CAD build for the part. Positions are in the model's coordinates, mm. Face numbers are marked on the shaded views. A direction names the side the tool comes from. Coordinates: 2 decimals unless noted, no trailing zeros. Loops run counter-clockwise (first coordinate to the right, second up) from the corner with the lowest first, then second, coordinate; pieces in that order, holes last. Notation, with made-up numbers: (4, -3) -> (21, -3) arc R27 cw to (21, 27) -> close; hole circle Ø4 at (77, 86). An arc over 180 degrees is marked (long way). Return JSON: item names as keys, results as strings. Group by question number.
(1) Flat gauge pins, fed straight in: pin 1 Ø0.8 at (y, z) = (-199, 56.5) entering from +X; pin 2 Ø0.5 at (x, z) = (150.5, 36) entering from -Y; pin 3 Ø6 at (x, z) = (86, 46) entering from -Y; pin 4 Ø1.1 at (y, z) = (0.5, 36) entering from -X. Where does each tip first touch, or does it go through?
(2) Saw through at D-D on x = -201. Write the cut outline in (y, z), then the cut area to 3 significant figures.
(3) Saw through at C-C on y = 153. Write the cut outline in (x, z), then the cut area to 3 significant figures.
(4) Saw through at A-A on z = 51.5. Write the cut outline in (x, y), then the cut area to 3 significant figures.
(5) Saw through at B-B on x = -31. Write the cut outline in (y, z).
(6) Probe L1, parallel to Y at x = -49.5, z = 43.25; L2, parallel to Y at x = -190, z = 54; L3, parallel to Z at x = -160.5, y = 91. List the from-to ranges inside material, lowest first.
(7) Tool access for the marked faces 5 and 6: list every direction of +Z, -Z, +X, -X, +Y, -Y with a clear straight run to the whole face (end or side of a thin tool).
(8) Mould opens along Y. For the marked faces 1, 2, 3 and 4 say: pulls with the +Y half, pulls with the -Y half, needs draft (parallel to the pull), parting line crosses it, or undercut.
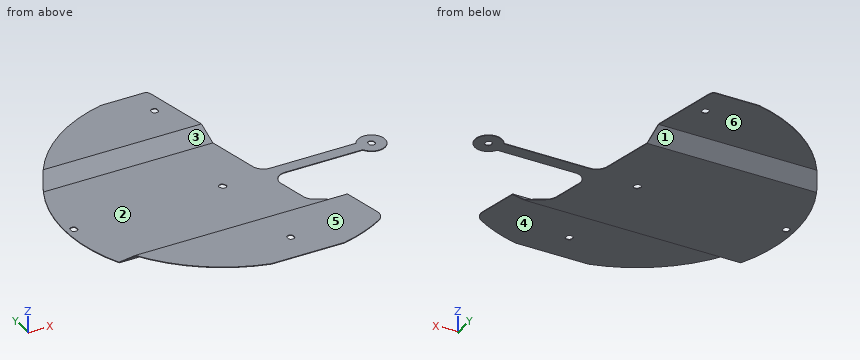
```python
from build123d import *

# Parameters (mm, degrees)
SALIENTE_EXTRUIR1_DEPTH    = 271
CORTAR_EXTRUIR6_DEPTH      = 372.705950862
CORTAR_EXTRUIR6_DEPTH_BACK = 372.705950862
CROQUIS2_W                 = 769.435607064
CROQUIS2_H                 = 651.661171996
CORTAR_EXTRUIR9_DEPTH      = 367.633759911
CORTAR_EXTRUIR9_DEPTH_BACK = 367.633759911


with BuildPart() as part:
    # Croquis1 → Saliente-Extruir1 (new, symmetric)
    with BuildSketch(Plane(origin=(0, 0, 0), x_dir=(0, 0, -1), z_dir=(1, 0, 0))):
        Polygon((-36.5, -110), (-36.5, 110), (-56.747809705, 134.130399958), (-56.747809705, 248), (-55.747809705, 248), (-55.747809705, 134.494370193), (-35.5, 110.363970234), (-35.5, -110.363970234), (-55.747809705, -134.494370193), (-55.747809705, -248), (-56.747809705, -248), (-56.747809705, -134.130399958), align=None)
    extrude(amount=SALIENTE_EXTRUIR1_DEPTH, both=True)

    # Croquis2 → Cortar-Extruir6 (cut, two sides: drawn at the far end of the back side and taken through both)
    with BuildSketch(Plane.XY.offset(-CORTAR_EXTRUIR6_DEPTH_BACK)):
        Rectangle(CROQUIS2_W, CROQUIS2_H)
        with BuildLine():
            ThreePointArc((18.264078831, 239.138091094), (11.247490428, 250.568826506), (-1.413221116, 254.996083903))
            ThreePointArc((-1.413221116, 254.996083903), (-245.428142449, -69.210020185), (132.017150423, -218.166156849))
            ThreePointArc((132.017150423, -218.166156849), (140.013145358, -209.009152502), (141.22932319, -196.913385678))
            Line((141.22932319, -196.913385678), (124.678167335, -118.72145722))
            ThreePointArc((124.678167335, -118.72145722), (121.297013967, -111.114290122), (115.11170826, -105.54264919))
            Line((115.11170826, -105.54264919), (95.618429873, -94.288199666))
            ThreePointArc((95.618429873, -94.288199666), (89.433124166, -88.716558735), (86.051970798, -81.109391636))
            Line((86.051970798, -81.109391636), (76.110157122, -34.141700046))
            ThreePointArc((76.110157122, -34.141700046), (80.139016625, -17.407025787), (95.676616197, -10))
            Line((95.676616197, -10), (222.404082058, -10))
            ThreePointArc((222.404082058, -10), (264, 0), (222.404082058, 10))
            Line((222.404082058, 10), (82.976208739, 10))
            ThreePointArc((82.976208739, 10), (70.383234525, 14.462400428), (63.409749664, 25.858299954))
            Line((63.409749664, 25.858299954), (18.264078831, 239.138091094))
        make_face(mode=Mode.SUBTRACT)
    extrude(amount=CORTAR_EXTRUIR6_DEPTH + CORTAR_EXTRUIR6_DEPTH_BACK, mode=Mode.SUBTRACT)

    # Croquis4 → Cortar-Extruir9 (cut, two sides: drawn at the far end of the back side and taken through both)
    with BuildSketch(Plane.XY.offset(-CORTAR_EXTRUIR9_DEPTH_BACK)):
        with BuildLine():
            Line((-5, 201.31662479), (-5, 194.68337521))
            ThreePointArc((-5, 194.68337521), (0, 192), (5, 194.68337521))
            Line((5, 194.68337521), (5, 201.31662479))
            ThreePointArc((5, 201.31662479), (0, 204), (-5, 201.31662479))
        make_face()
        with BuildLine():
            Line((5, -201.31662479), (5, -194.68337521))
            ThreePointArc((5, -194.68337521), (0, -192), (-5, -194.68337521))
            Line((-5, -194.68337521), (-5, -201.31662479))
            ThreePointArc((-5, -201.31662479), (0, -204), (5, -201.31662479))
        make_face()
        with BuildLine():
            Line((-247, 3.31662479), (-247, -3.31662479))
            ThreePointArc((-247, -3.31662479), (-242, -6), (-237, -3.31662479))
            Line((-237, -3.31662479), (-237, 3.31662479))
            ThreePointArc((-237, 3.31662479), (-242, 6), (-247, 3.31662479))
        make_face()
        with BuildLine():
            Line((237, 3.31662479), (237, -3.31662479))
            ThreePointArc((237, -3.31662479), (242, -6), (247, -3.31662479))
            Line((247, -3.31662479), (247, 3.31662479))
            ThreePointArc((247, 3.31662479), (242, 6), (237, 3.31662479))
        make_face()
        with BuildLine():
            Line((-5.933205139, 0.892791565), (-3.129872731, -5.118974183))
            ThreePointArc((-3.129872731, -5.118974183), (2.53570957, -5.437846722), (5.933205139, -0.892791565))
            Line((5.933205139, -0.892791565), (3.129872731, 5.118974183))
            ThreePointArc((3.129872731, 5.118974183), (-2.53570957, 5.437846722), (-5.933205139, 0.892791565))
        make_face()
    extrude(amount=CORTAR_EXTRUIR9_DEPTH + CORTAR_EXTRUIR9_DEPTH_BACK, mode=Mode.SUBTRACT)


solid = part.part
```
Geometry results:
{
 "1": {"pin 1": "x = 141.59", "pin 2": "y = -10", "pin 3": "y = -126.45", "pin 4": "x = -255"},
 "2": {"outline": "(-156.92, 55.75) -> (-134.49, 55.75) -> (-110.36, 35.5) -> (110.36, 35.5) -> (134.49, 55.75) -> (156.92, 55.75) -> (156.92, 56.75) -> (134.13, 56.75) -> (110, 36.5) -> (-110, 36.5) -> (-134.13, 56.75) -> (-156.92, 56.75) -> close", "area": "329 mm²"},
 "3": {"outline": "(-204, 55.75) -> (36.5, 55.75) -> (36.5, 56.75) -> (-204, 56.75) -> close", "area": "240 mm²"},
 "4": {"outline": "(-220.62, -127.88) arc R255 ccw to (-219.71, -129.43) -> (126.95, -129.43) -> (126.62, -127.88) -> close; (-220.62, 127.88) -> (41.82, 127.88) -> (41.49, 129.43) -> (-219.71, 129.43) arc R255 ccw to start", "area": "947 mm²"},
 "5": {"outline": "(-248, 55.75) -> (-134.49, 55.75) -> (-110.36, 35.5) -> (110.36, 35.5) -> (134.49, 55.75) -> (248, 55.75) -> (248, 56.75) -> (134.13, 56.75) -> (110, 36.5) -> (-110, 36.5) -> (-134.13, 56.75) -> (-248, 56.75) -> close"},
 "6": {"L1": "-119.6 to -118.04, 118.04 to 119.6", "L2": "-132.41 to -130.86, 130.86 to 132.41", "L3": "35.5 to 36.5"},
 "7": {"face 5": "+Z, +X, -X, +Y, -Y", "face 6": "-Z, +X, -X, +Y"},
 "8": {"face 1": "pulls with the +Y half", "face 2": "undercut", "face 3": "undercut", "face 4": "needs draft"}
}
